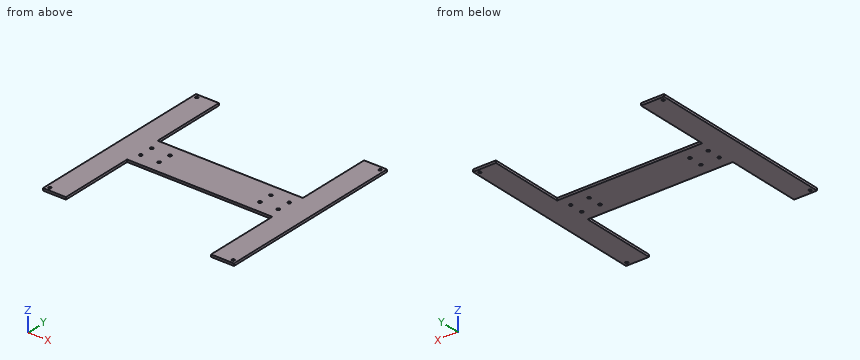
from build123d import *

# Parameters (mm, degrees)
SKETCH1_R           = 2
BOSS_EXTRUDE1_DEPTH = 3
SKETCH3_R           = 1.75
CUT_EXTRUDE1_DEPTH  = 3


with BuildPart() as part:
    # Sketch1 → Boss-Extrude1 (new body)
    with BuildSketch(Plane.XY):
        Polygon((95, 125), (125, 125), (125, -125), (95, -125), (95, -25), (-95, -25), (-95, -125), (-125, -125), (-125, 125), (-95, 125), (-95, 25), (95, 25), align=None)
        with Locations((90, 9)):
            Circle(SKETCH1_R, mode=Mode.SUBTRACT)
        with Locations((90, -9)):
            Circle(SKETCH1_R, mode=Mode.SUBTRACT)
        with Locations((66, 9)):
            Circle(SKETCH1_R, mode=Mode.SUBTRACT)
        with Locations((66, -9)):
            Circle(SKETCH1_R, mode=Mode.SUBTRACT)
        with Locations((-66, -9)):
            Circle(SKETCH1_R, mode=Mode.SUBTRACT)
        with Locations((-66, 9)):
            Circle(SKETCH1_R, mode=Mode.SUBTRACT)
        with Locations((-90, -9)):
            Circle(SKETCH1_R, mode=Mode.SUBTRACT)
        with Locations((-90, 9)):
            Circle(SKETCH1_R, mode=Mode.SUBTRACT)
    extrude(amount=BOSS_EXTRUDE1_DEPTH)

    # Sketch3 → Cut-Extrude1 (cut)
    with BuildSketch(Plane.XY.offset(3)):
        with Locations((-120, 120)):
            Circle(SKETCH3_R)
        with Locations((120, 120)):
            Circle(SKETCH3_R)
        with Locations((-120, -120)):
            Circle(SKETCH3_R)
        with Locations((120, -120)):
            Circle(SKETCH3_R)
    extrude(amount=-CUT_EXTRUDE1_DEPTH, mode=Mode.SUBTRACT)


solid = part.part
Geometry: final body of the model. Coordinates: model frame, mm. Give positions to 0.01 mm unless a question says otherwise; leave off trailing zeros. Write each loop counter-clockwise with the first axis right and the second up, starting at its lowest first coordinate (ties: lowest second). Pieces come first, ordered by that corner, then holes.
(1) Ray query, line 1 (Y direction, x = -120, z = 1.7); line 2 (Y direction, x = 66, z = 1); line 3 (X direction, y = -120, z = 0.7). Return the intervals inside material, ascending.
(2) Cut plane B-B, the plane z = 1.05. Give the number of separate pieces and of enclosed holes in the cut face, then the cut area to 3 significant figures.
(3) First-contact query: P1, Ø1.5, axis at x = -18, z = 0.5, coming from the -Y side; P2, Ø2, axis at x = -120, y = -120, coming from the -Z side; P3, Ø0.9, axis at x = -29, z = 1, coming from the +Y side. Flat tips, straight axial feed; report the tip coordinate or a pass-through.
(4) Cut plane C-C, the plane x = -8.5. Return loops of the section in (y, z), then the cut area to 3 significant figures.
(5) Cut plane A-A, the plane y = -97.5. Return loops of the section in (x, z), then the cut area to 3 significant figures.
Values follow:
1. line 1: y = -125 to -121.75, -118.25 to 118.25, 121.75 to 125
1. line 2: y = -25 to -11, -7 to 7, 11 to 25
1. line 3: x = -125 to -121.75, -118.25 to -95, 95 to 118.25, 121.75 to 125
2. separate pieces: 1
2. enclosed holes: 12
2. area: 24,400 mm2
3. P1: stops at y = -25
3. P2: passes through
3. P3: stops at y = 25
4. outline: (-25, 0) - (25, 0) - (25, 3) - (-25, 3) - close
4. area: 150 mm2
5. outline: (-125, 0) - (-95, 0) - (-95, 3) - (-125, 3) - close; (95, 0) - (125, 0) - (125, 3) - (95, 3) - close
5. area: 180 mm2
